Autodesk Fusion 360 part; units mm, degrees
sketch "Front Face" plane through (0, 0, 0) normal (0, 1, 0) x (1, 0, 0)
  line L0 (4.5, 12) -> (-4.5, 12)
  line L1 (-4.5, 12) -> (-4.5, -12)
  line L2 (-4.5, -12) -> (4.5, -12)
  line L3 (4.5, -12) -> (4.5, 12)
  line L4 (4.5, 12) -> (-4.5, -12) construction
  line L5 (-4.5, 12) -> (4.5, -12) construction
  circle A0 centre (0, 6) radius 3.15
  line L6 (3.4751, 1) -> (-3.4751, 1)
  line L7 (-3.4751, 1) -> (-3.4751, -10.5)
  line L8 (-3.4751, -10.5) -> (3.4751, -10.5)
  line L9 (3.4751, -10.5) -> (3.4751, 1)
  line L10 (3.4751, 1) -> (-3.4751, -10.5) construction
  line L11 (-3.4751, 1) -> (3.4751, -10.5) construction
  circle A1 centre (0, 6) radius 1.05
  line L12 (0, -12) -> (0, 12) construction
  circle A2 centre (0, -1.9607) radius 1.75
  circle A3 centre (0, -1.9607) radius 1.25
  line L13 (0.25, -6.0814) -> (-0.25, -6.0814)
  line L14 (-0.25, -6.0814) -> (-0.25, -9.0814)
  line L15 (-0.25, -9.0814) -> (0.25, -9.0814)
  line L16 (0.25, -9.0814) -> (0.25, -6.0814)
  line L17 (0.25, -6.0814) -> (-0.25, -9.0814) construction
  line L18 (-0.25, -6.0814) -> (0.25, -9.0814) construction
  point P0 (0, -4.75)
  point P1 (0, -7.5814)
  dimension "d1" = 24
  dimension "d2" = 9
  dimension "d3" = 6.3
  dimension "d4" = 1.5
  dimension "d5" = 1
  dimension "d6" = 6
  dimension "d11" = 2.1
  dimension "d12" = 0.5
  dimension "d13" = 2.5
  dimension "d14" = 0.5
  dimension "d15" = 3
extrude "Extrude1" add sketch "Front Face" along normal blind 14.1 contours L0 L1 L2 L3 | A0 | L6 L7 L8 L9 | A1 | A2 | A3 | L13 L14 L15 L16
extrude "Extrude2" cut sketch "Front Face" along normal blind 10 contours A0
extrude "Extrude3" cut sketch "Front Face" along normal blind 1 contours L6 L7 L8 L9 | A3
chamfer "Chamfer1" distance 0.8 distance2 2 1 edges at (-0.9789, 0, -6.3797) measured on face at (0.3381, 0, -5.6969)
fillet "Fillet1" radius 0.4 6 edges at (4.5, 0, 0) (0, 0, 12) (-4.5, 0, 0) (0, 0, -12) (4.5, 7.05, 12) (-4.5, 7.05, 12)
sketch "Bottom Lugs" plane through (0, 0, -12) normal (0, 0, -1) x (1, 0, 0)
  line L0 (4.5, -0.4) -> (-4.5, -0.4)
  line L1 (-4.5, -0.4) -> (-4.5, -14.1)
  line L2 (-4.5, -14.1) -> (4.5, -14.1)
  line L3 (4.5, -14.1) -> (4.5, -0.4)
  line L4 (-1.2, -7.195) -> (1.2, -7.195)
  line L5 (1.2, -7.195) -> (1.2, -7.445)
  line L6 (1.2, -7.445) -> (-1.2, -7.445)
  line L7 (-1.2, -7.445) -> (-1.2, -7.195)
  line L8 (4.5, -8.985) -> (4.9, -8.985)
  line L9 (4.9, -8.985) -> (4.9, -11.335)
  line L10 (4.9, -11.335) -> (4.5, -11.335)
  line L11 (4.5, -11.335) -> (4.5, -8.985)
  line L12 (-1.65, -13.1) -> (1.2, -13.1)
  line L13 (1.2, -13.1) -> (1.2, -13.5)
  line L14 (1.2, -13.5) -> (-1.65, -13.5)
  line L15 (-1.65, -13.5) -> (-1.65, -13.1)
  line L16 (4.5, 0) -> (-4.5, 0)
  point P0 (0, -7.195)
  point P1 (1.2, -7.32)
  point P2 (1.2, -13.3)
  point P3 (4.7, -11.335)
  point P4 (4.9, -10.16)
  dimension "d21" = 0.25
  dimension "d22" = 2.4
  dimension "d23" = 0.4
  dimension "d24" = 2.35
  dimension "d25" = 2.85
  dimension "d26" = 0.4
  dimension "d28" = 7.32
  dimension "d29" = 13.3
  dimension "d30" = 4.7
  dimension "d33" = 10.16
extrude "Extrude4" add sketch "Bottom Lugs" along normal blind 3.8 contours L4 L5 L6 L7 | L12 L13 L14 L15
extrude "Extrude5" add sketch "Bottom Lugs" along normal mid plane 7.6 contours L3 L8 L9 L10 L11
fillet "Fillet2" radius 1.175 4 edges at (4.7, 8.985, -15.8) (4.7, 11.335, -15.8) (4.7, 8.985, -8.2) (4.7, 11.335, -8.2)
fillet "Fillet2" radius 1.425 2 edges at (1.2, 13.3, -15.8) (-1.65, 13.3, -15.8)
fillet "Fillet2" radius 1.2 2 edges at (1.2, 7.32, -15.8) (-1.2, 7.32, -15.8)
hole "Hole1" at (0, 7.195, -14.6) direction (0, 1, 0) diameter 1 depth 1 tip angle 180
hole "Hole2" at (-0.225, 13.1, -14.375) direction (0, 1, 0) diameter 1.5 depth 1.5 tip angle 180
hole "Hole3" at (4.9, 10.16, -14.625) direction (-1, 0, 0) diameter 1 depth 1 tip angle 180
sketch "Sketch3" plane through (0, 0, 12) normal (0, 0, 1) x (-1, 0, 0)
  line L0 (4.1, -14.1) -> (4.1, -0.4)
  line L1 (4.1, -0.4) -> (-4.1, -0.4)
  line L2 (-4.1, -0.4) -> (-4.1, -14.1)
  line L3 (-4.1, -14.1) -> (4.1, -14.1)
  line L4 (4.5, -0.4) -> (4.5, -14.1)
  line L5 (-4.5, -14.1) -> (-4.5, -0.4)
  line L6 (4.5, -8.8) -> (-4.5, -8.8)
  line L7 (-4.5, -8.8) -> (-4.5, -1)
  line L8 (-4.5, -1) -> (4.5, -1)
  line L9 (4.5, -1) -> (4.5, -8.8)
  line L10 (-4.5, 0) -> (4.5, 0)
  dimension "d48" = 1
  dimension "d49" = 8.8
extrude "Extrude6" cut sketch "Sketch3" against normal blind 0.5 contours L0 L2 L6 L8 | L0 L4 L6 L8 L9 | L2 L5 L6 L7 L8
extrude "Extrude7" cut sketch "Sketch3" against normal blind 9.25 contours L0 L4 L6 L8 L9 | L2 L5 L6 L7 L8
equation "d36 = ( 2.35 / 2 ) * 1 mm"
equation "d37 = ( 2.85 / 2 ) * 1 mm"
equation "d38 = ( 2.4 / 2 ) * 1 mm"
equation "d52 = -18.5 mm / 2"

Autodesk Fusion 360 part; units mm, degrees
box "BoxPrimitive1" add length 62.5 width 22 height 13.25 placed x (0, 1, 0) y (-1, 0, 0) z (0, 0, 1) at (22, 0, 0)
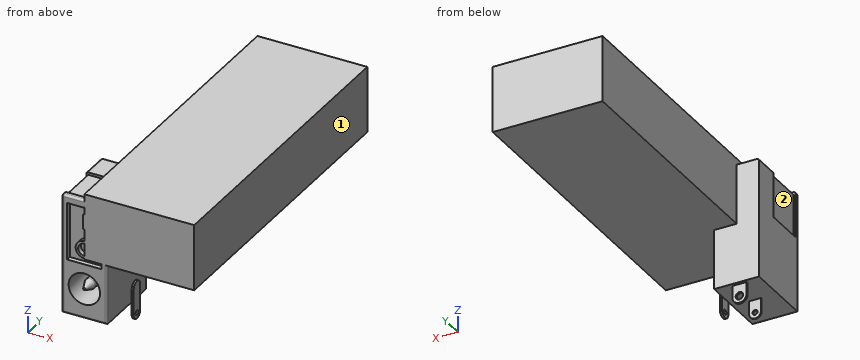
Build history of the part. All positions in model axes, mm. Face numbers are marked on the shaded views. A direction names the side the tool comes from. Coordinates: 2 decimals unless noted, no trailing zeros. Write each loop counter-clockwise with the first axis right and the second up, starting at its lowest first coordinate (ties: lowest second). Pieces come first, ordered by that corner, then holes.
(1) Cut at B-B on z = -10.5. List the corners of the cut face in (x, y) (3 decimals), and give its area (3 significant figures).
(2) 3-axis set-ups, long thin cutter, end or side, ignore diameter. For the marked faces 1 and 2: which of +Z, -Z, +X, -X, +Y, -Y reach the whole face in a straight line?
(3) Pin check, flat tips, straight feed: pin 1 Ø3 at (x, y) = (9, 30) entering from -Z; pin 2 Ø2 at (x, z) = (-3, 8) entering from +Y; pin 3 Ø1.2 at (y, z) = (10.5, -11.5) entering from +X. Stop position of each tip, or through.
(4) Cut at C-C on x = 12. List the corners of the cut face in (y, z).
(5) Cut at A-A on z = 7.5. List the corners of the cut face in (x, y).
(6) Drill centre lines: line 1 (Z direction, x = 4.75, y = 10.16) (3 decimals); line 2 (Z direction, x = 2, y = 40.5); line 3 (Y direction, x = -1, z = 3.75). Where is each one in solid material? Low to high.
(7) Cut at D-D on y = 51. List the corners of the cut face in (x, z), and give its area (4 significant figures).
Working result:
1. outline: (-4.5, 0.4) arc R0.4 ccw to (-4.1, 0) - (4.1, 0) arc R0.4 ccw to (4.5, 0.4) - (4.5, 8.985) - (4.9, 8.985) - (4.9, 11.335) - (4.5, 11.335) - (4.5, 14.1) - (-4.5, 14.1) - close
1. area: 128 mm2
2. face 1: +Z, -Z, +X, +Y, -Y
2. face 2: +Z, -X
3. pin 1: stops at z = 0
3. pin 2: stops at y = 14.1
3. pin 3: stops at x = 4.9
4. outline: (0, 0) - (62.5, 0) - (62.5, 13.25) - (0, 13.25) - close
5. outline: (-4.5, 0.4) arc R0.4 ccw to (-4.1, 0) - (-3.48, 0) - (-3.48, 1) - (-0.25, 1) - (-0.25, 0) - (22, 0) - (22, 62.5) - (0, 62.5) - (0, 14.1) - (-4.5, 14.1) - (-4.5, 8.8) - (-4.1, 8.8) - (-4.1, 1) - (-4.5, 1) - close
6. line 1: z = -15.8 to -15.125, -14.125 to -8.2, 0 to 13.25
6. line 2: z = 0 to 13.25
6. line 3: y = 1 to 14.1
7. outline: (0, 0) - (22, 0) - (22, 13.25) - (0, 13.25) - close
7. area: 291.5 mm2
